Drawing for the job (mm, zero at the part's lowest x, y, z). A direction names the side the tool comes from. Coordinates: 2 decimals unless noted, no trailing zeros. Loops run counter-clockwise (first coordinate to the right, second up) from the corner with the lowest first, then second, coordinate; pieces in that order, holes last. Notation, with made-up numbers: (-16.75, 86) - (21.25, 86) arc R32 ccw to (21.25, 123) - close; hole circle Ø10 at (88, 58.5). An arc over 180 degrees is marked (long way). Put each result on its own line as item: value.
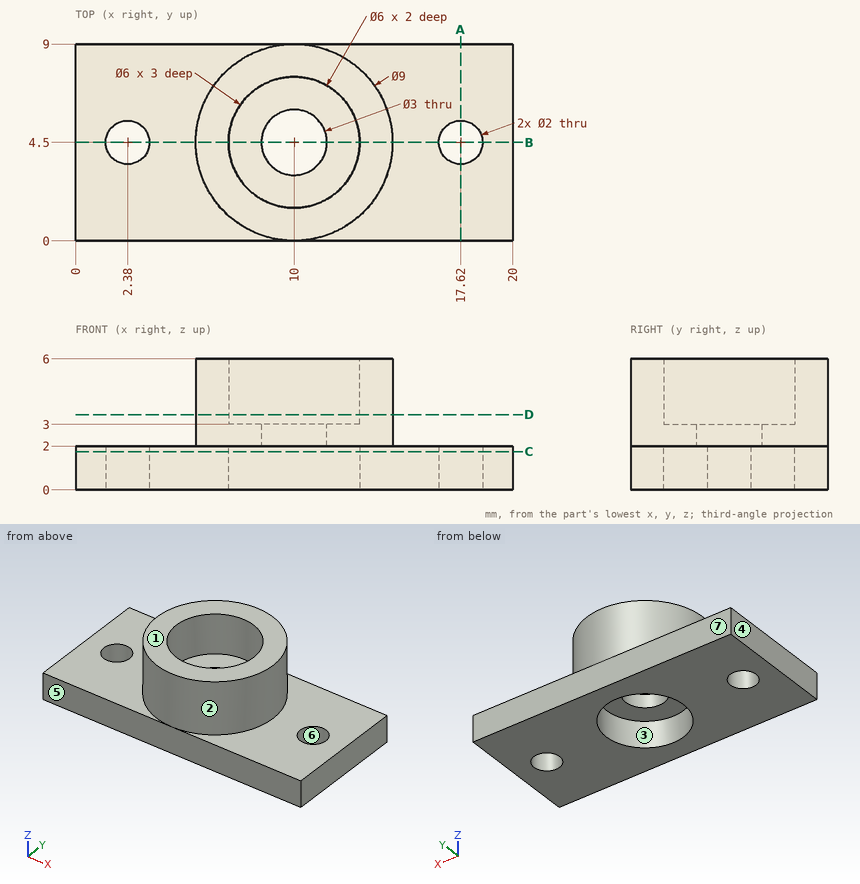
Q1. Slice it at C-C, the plane z = 1.75. Give the cut face in (x, y).
Determined:
outline: (0, 0) - (20, 0) - (20, 9) - (0, 9) - close; hole circle Ø2 at (2.38, 4.5); hole circle Ø6 at (10, 4.5); hole circle Ø2 at (17.62, 4.5)
Q2. Pin check, flat tips, straight feed: pin 1 Ø3.5 at (x, y) = (10, 4.5) entering from +Z; pin 2 Ø1.2 at (x, y) = (2.38, 4.5) entering from -Z; pin 3 Ø2.5 at (x, y) = (17.62, 4.5) entering from +Z; pin 4 Ø1.5 at (x, z) = (12, 3) entering from -Y. Stop position of each tip, or through.
Determined:
pin 1: z = 3
pin 2: through
pin 3: z = 2
pin 4: y = 0.18
Q3. Tool access for the marked faces 1, 2 and 3: list every direction of +Z, -Z, +X, -X, +Y, -Y with a clear straight run to the whole face (end or side of a thin tool).
Determined:
face 1: +Z, +X, -X, +Y, -Y
face 2: +Z
face 3: -Z
Q4. Slice it at A-A, the plane x = 17.62. Give the cut face in (y, z).
Determined:
outline: (0, 0) - (3.5, 0) - (3.5, 2) - (0, 2) - close; (5.5, 0) - (9, 0) - (9, 2) - (5.5, 2) - close
Q5. Wall check: L1, parallel to Y at x = 10, z = 5.3; L2, parallel to Y at x = 10, z = 2.5; L3, parallel to Z at x = 2.5, y = 7. Give the ranges that are in metal, low to high. Write a range as from..to.
Determined:
L1: 0..1.5, 7.5..9
L2: 0..3, 6..9
L3: 0..2
Q6. Mould opens along Y. For the marked faces 4, 5, 6 and 7 say: +Y half, -Y half, draft (parallel to the pull), parting line (faces both ways), or undercut.
Determined:
face 4: draft
face 5: -Y half
face 6: undercut
face 7: +Y half
Q7. Slice it at D-D, the plane z = 3.45. Give the cut face in (x, y).
Determined:
outline: circle Ø9 at (10, 4.5); hole circle Ø6 at (10, 4.5)
Q8. Slice it at B-B, the plane y = 4.5. Give the cut face in (x, z), then the cut area to 3 significant figures.
Determined:
outline: (0, 0) - (1.38, 0) - (1.38, 2) - (0, 2) - close; (3.38, 0) - (7, 0) - (7, 2) - (8.5, 2) - (8.5, 3) - (7, 3) - (7, 6) - (5.5, 6) - (5.5, 2) - (3.38, 2) - close; (11.5, 2) - (13, 2) - (13, 0) - (16.62, 0) - (16.62, 2) - (14.5, 2) - (14.5, 6) - (13, 6) - (13, 3) - (11.5, 3) - close; (18.62, 0) - (20, 0) - (20, 2) - (18.62, 2) - close
area: 35.0 mm2
